Autodesk Inventor part; units mm, degrees
ref_plane "YZ Plane" through (0, 0, 0) normal (1, 0, 0) x (0, 1, 0)
ref_plane "XZ Plane" through (0, 0, 0) normal (0, 1, 0) x (-1, 0, 0)
ref_plane "XY Plane" through (0, 0, 0) normal (0, 0, 1) x (1, 0, 0)
sketch "Sketch1" plane through (0, 0, 0) normal (0, 0, 1) x (1, 0, 0)
  line L0 (66, -34) -> (-66, -34)
  line L1 (-66, -34) -> (-66, 34)
  line L2 (-66, 34) -> (66, 34)
  line L3 (66, 34) -> (66, -34)
  line L4 (66, -34) -> (-66, 34) construction
  line L5 (-66, -34) -> (66, 34) construction
  line L6 (74, 42) -> (-74, 42)
  line L7 (-74, 42) -> (-74, -42)
  line L8 (-74, -42) -> (74, -42)
  line L9 (74, -42) -> (74, 42)
  line L10 (-74, 38) -> (-89, 38)
  line L11 (-97.5, 29.5) -> (-97.5, 10.5)
  line L12 (-89, 2) -> (-66, 2)
  line L13 (-66, 2) -> (-66, 34)
  line L14 (74, -38) -> (89, -38)
  line L15 (97.5, -29.5) -> (97.5, -10.5)
  line L16 (89, -2) -> (66, -2)
  line L17 (66, -2) -> (66, -34)
  line L18 (-89, 29.5) -> (-89, 10.5) construction
  line L19 (-83, 29.5) -> (-83, 10.5)
  line L20 (-95, 10.5) -> (-95, 29.5)
  arc A0 (-83, 29.5) -> (-95, 29.5) centre (-89, 29.5) ccw
  arc A1 (-95, 10.5) -> (-83, 10.5) centre (-89, 10.5) ccw
  arc A2 (-89, 38) -> (-97.5, 29.5) centre (-89, 29.5) ccw
  arc A3 (-97.5, 10.5) -> (-89, 2) centre (-89, 10.5) ccw
  line L21 (89, -10.5) -> (89, -29.5) construction
  line L22 (83, -10.5) -> (83, -29.5)
  line L23 (95, -29.5) -> (95, -10.5)
  arc A4 (95, -10.5) -> (83, -10.5) centre (89, -10.5) ccw
  arc A5 (83, -29.5) -> (95, -29.5) centre (89, -29.5) ccw
  arc A6 (97.5, -10.5) -> (89, -2) centre (89, -10.5) ccw
  arc A7 (89, -38) -> (97.5, -29.5) centre (89, -29.5) ccw
  line L24 (70.75, -38.75) -> (-70.75, -38.75) construction
  line L25 (-70.75, -38.75) -> (-70.75, 38.75) construction
  line L26 (-70.75, 38.75) -> (70.75, 38.75) construction
  line L27 (70.75, 38.75) -> (70.75, -38.75) construction
  line L28 (70.75, -38.75) -> (-70.75, 38.75) construction
  line L29 (-70.75, -38.75) -> (70.75, 38.75) construction
  line L30 (89, -10.5) -> (89, 8.5) construction
  line L31 (83, -10.5) -> (83, 8.5)
  line L32 (95, 8.5) -> (95, -10.5)
  arc A8 (83, -10.5) -> (95, -10.5) centre (89, -10.5) ccw
  arc A9 (95, 8.5) -> (83, 8.5) centre (89, 8.5) ccw
  line L33 (66, 17) -> (89, 17)
  line L34 (97.5, 8.5) -> (97.5, -10.5)
  arc A10 (97.5, 8.5) -> (89, 17) centre (89, 8.5) ccw
  point P0 (0, 0)
  point P1 (-89, 20)
  point P2 (89, -20)
  point P3 (-74, 2)
  point P4 (74, -38.3314)
  point P5 (74, -2)
  point P6 (-74, 37.5)
  point P7 (-70.75, 20)
  point P8 (-70.75, 0)
  point P9 (-70.75, -20)
  point P10 (-37.446, 41.825)
  point P11 (-13.2416, 41.825)
  point P12 (11.1286, 41.825)
  point P13 (33.3436, 41.825)
  point P14 (70.75, 20)
  point P15 (70.75, 0)
  point P16 (70.75, -20)
  point P17 (-20, -38.75)
  point P18 (-40, -38.75)
  point P19 (-5.5184, 38.75)
  point P20 (-70.75, -13.3991)
  point P21 (70.75, 0)
  point P22 (0, -38.75)
  point P23 (-60, -38.75)
  point P24 (0, -38.75)
  point P25 (89, -1)
  point P26 (74, 17)
  dimension "d0" = 132
  dimension "d1" = 68
  dimension "d2" = 8
  dimension "d5" = 6
  dimension "d6" = 19
  dimension "d8" = 2.5
  dimension "d9" = 15
  dimension "d11" = 2.5
  dimension "d12" = 15
  dimension "d17" = 20
  dimension "d21" = 20
  dimension "d22" = 20
  dimension "d32" = 3.25
  dimension "d33" = 3.25
  dimension "d36" = 20
  dimension "d37" = 20
  dimension "d38" = 18.75
extrude "Extrusion1" add sketch "Sketch1" along normal blind 1.6 contours L3 L16 L9 L8 L7 L12 L1 L0 | L0 L1 L2 L3 | L3 L33 L9 L16 | L12 L7 L6 L9 L33 L3 L2 L1 | L16 L31 L22 A5 L23 L32 A6 L15 A7 L14 L9 | L12 A3 L11 A2 L10 L7 | L16 A6 L32 A4 L31 | A8 L23 A5 L22 | A4 A8 | L19 A1 L20 A0
hole "Hole1" at (-70.75, 0, 0) at (-70.75, -20, 0) at (-20, -38.75, 0) at (-40, -38.75, 0) at (0, -38.75, 0) at (-60, -38.75, 0) direction (0, 0, 1) diameter 3.2 end through all
mirror "Mirror1" about plane through (0, 0, 0) normal (1, 0, 0) of "Hole1"
mirror "Mirror2" about plane through (0, 0, 0) normal (0, 1, 0) of "Hole1", "Mirror1"
extrude "Extrusion2" add sketch "Sketch1" along normal up to surface (1.6 mm away) contours L9 L33 A10 L34 A6 L32 A9 L31 L16 | L31 A9 L32 A6 L16
fillet "Fillet1" radius 2 4 edges at (-74, -42, 0.8) (74, -42, 0.8) (74, 42, 0.8) (-74, 42, 0.8)
fillet "Fillet2" radius 2 4 edges at (-74, 2, 0.8) (-74, 38, 0.8) (74, -38, 0.8) (74, 17, 0.8)
sketch "Sketch2" plane through (0, 0, 1.6) normal (0, 0, 1) x (1, 0, 0)
  arc A0 (-72, 42) -> (-74, 40) centre (-72, 40) ccw
  line L0 (-74, 0) -> (-74, -40)
  arc A1 (-76, 38) -> (-74, 40) centre (-76, 40) ccw
  line L1 (-76, 38) -> (-89, 38)
  arc A2 (-89, 38) -> (-97.5, 29.5) centre (-89, 29.5) ccw
  line L2 (-97.5, 29.5) -> (-97.5, 10.5)
  arc A3 (-97.5, 10.5) -> (-89, 2) centre (-89, 10.5) ccw
  line L3 (-89, 2) -> (-76, 2)
  arc A4 (-74, 0) -> (-76, 2) centre (-76, 0) ccw
  arc A5 (-74, -40) -> (-72, -42) centre (-72, -40) ccw
  line L4 (-72, -42) -> (72, -42)
  arc A6 (72, -42) -> (74, -40) centre (72, -40) ccw
  line L5 (74, 19) -> (74, 40)
  arc A7 (76, -38) -> (74, -40) centre (76, -40) ccw
  line L6 (76, -38) -> (89, -38)
  arc A8 (89, -38) -> (97.5, -29.5) centre (89, -29.5) ccw
  line L7 (97.5, -29.5) -> (97.5, 8.5)
  arc A9 (74, 40) -> (72, 42) centre (72, 40) ccw
  line L8 (72, 42) -> (-72, 42)
  circle A10 centre (60, 38.75) radius 1.6
  circle A11 centre (70.75, 20) radius 1.6
  circle A12 centre (20, 38.75) radius 1.6
  circle A13 centre (40, 38.75) radius 1.6
  circle A14 centre (-60, 38.75) radius 1.6
  circle A15 centre (-70.75, 20) radius 1.6
  circle A16 centre (-20, 38.75) radius 1.6
  circle A17 centre (-40, 38.75) radius 1.6
  circle A18 centre (0, 38.75) radius 1.6
  circle A19 centre (60, -38.75) radius 1.6
  circle A20 centre (70.75, 0) radius 1.6
  circle A21 centre (70.75, -20) radius 1.6
  circle A22 centre (20, -38.75) radius 1.6
  circle A23 centre (40, -38.75) radius 1.6
  circle A24 centre (-60, -38.75) radius 1.6
  circle A25 centre (0, -38.75) radius 1.6
  circle A26 centre (-40, -38.75) radius 1.6
  circle A27 centre (-20, -38.75) radius 1.6
  circle A28 centre (-70.75, -20) radius 1.6
  circle A29 centre (-70.75, 0) radius 1.6
  arc A30 (97.5, 8.5) -> (89, 17) centre (89, 8.5) ccw
  line L9 (76, 17) -> (89, 17)
  arc A31 (74, 19) -> (76, 17) centre (76, 19) ccw
  point P0 (0, 0)
equation "\"d11\" = d8"
equation "\"d12\" = d9"
equation "\"d33\" = d32"
properties part number "Board Outline"
Read the model definition and answer for the solid it produces. Units are mm, in the model's axes. Round coordinates to 2 decimals unless told otherwise and drop trailing zeros. Order: outer loops, then holes, each group sorted by start corner. A loop starts at its lowest first (then second) coordinate and runs counter-clockwise, first axis right, second up. Notation, with made-up numbers: (6.5, -18) - (57.5, -18) arc R13 cw to (57.5, 7) - close; hole circle Ø9 at (50, 82.5). An arc over 180 degrees is marked (long way). Use one line per item in the form item = value. Start each with the question number.
(1) The part is cut by section A-A (z = 0.75). Count the separate pieces of the cut face and the enclosed holes in it, then the cut area to 3 significant figures.
(2) Flat-ended cylindrical pins translate along their axes: pin 1 Ø0.8 at (x, z) = (80, 1) entering from -Y; pin 2 Ø2.5 at (x, y) = (40, -38.75) entering from +Z. Find the tip coordinate at first contact, or state that the pin passes through.
(3) Determine the mould class of faces 1 (the face through (-1, 1, 1.6)), 2 (the face through (21.586, 38.958, 0.811)), 3 (the face through (94.94, 14.58, 0.79)) for opening direction Y: +Y half, -Y half, draft (parallel to the pull), parting line (faces both ways), or undercut.
(4) The part is cut by section B-B (y = -13.5). Give the vertices of the cut face in (x, z).
(5) Find the intervals of material crossed by line 1 along Y through (x, z) = (-60, 1.1); line 2 along X through (y, z) = (23, 1.15); line 3 along X through (y, z) = (-7.5, 0.8), in increasing order. Write a range as from..to.
(6) The part is cut by section C-C (y = -31.5). Give the vertices of the cut face in (x, z), then the cut area to 3 significant figures.
Checked values:
q1.separate_pieces = 1
q1.enclosed_holes = 20
q1.area = 14,300 mm^2
q2.pin_1 = -38
q2.pin_2 = through
q3.face_1 = draft
q3.face_2 = undercut
q3.face_3 = +Y half
q4.outline = (-74, 0) - (97.5, 0) - (97.5, 1.6) - (-74, 1.6) - close
q5.line_1 = -42..-40.35, -37.15..37.15, 40.35..42
q5.line_2 = -97.5..74
q5.line_3 = -74..97.5
q6.outline = (-74, 0) - (97.26, 0) - (97.26, 1.6) - (-74, 1.6) - close
q6.area = 274 mm^2
